The model under review builds one solid part; all positions refer to its coordinate system, in mm. Round coordinates to 2 decimals unless told otherwise and drop trailing zeros. Order: outer loops, then holes, each group sorted by start corner. A loop starts at its lowest first (then second) coordinate and runs counter-clockwise, first axis right, second up. Notation, with made-up numbers: (76, 49.5) - (84, 49.5) arc R14 cw to (84, 60.5) - close; hole circle Ø10 at (-2.75, -5). An arc over 180 degrees is marked (long way). One line per question, with ' | ' between items. Start each with the question number.
Item 1: Add section C-C on x = -2.5. State the section outline as (y, z) points.
Item 2: For L1, parallel to Z at x = -7.25, y = 20; L2, parallel to Z at x = -9.5, y = 20; L3, parallel to X at y = 25, z = 61, list the stretches that pass through material, from the lowest coordinate up. Write a range as [from, to].
Item 3: Add section D-D on z = -6. State the section outline as (x, y) points, and give its area (3 significant figures).
Item 4: Add section B-B on y = 12. State the section outline as (x, z) points, and give its area (3 significant figures).
Item 5: Add section A-A on y = 20. State the section outline as (x, z) points, and give its area (3 significant figures).
Item 6: Insertion check: pin 1 Ø3 at (x, y) = (-18, 15.5) entering from -Z; pin 2 Ø3 at (y, z) = (15, 62) entering from -X; pin 3 Ø10 at (x, y) = (-13, 34) entering from +Z; pin 4 Ø2.5 at (y, z) = (20, 11.74) entering from -X. Each pin has a flat end and moves straight along its axis. Give the tip position at first contact, or say it passes through.
Autodesk Inventor part; units mm, degrees
ref_plane "YZ Plane" through (0, 0, 0) normal (1, 0, 0) x (0, 1, 0)
ref_plane "XZ Plane" through (0, 0, 0) normal (0, 1, 0) x (-1, 0, 0)
ref_plane "XY Plane" through (0, 0, 0) normal (0, 0, 1) x (1, 0, 0)
sketch "Sketch1" plane through (0, 0, 0) normal (0, 1, 0) x (-1, 0, 0)
  line L0 (0.6887, 107.7362) -> (0.6887, -18.2638)
  line L1 (0.6887, -18.2638) -> (20.6887, 1.7362)
  line L2 (20.6887, 1.7362) -> (20.6887, 87.7362)
  line L3 (20.6887, 87.7362) -> (0.6887, 107.7362)
  point P0 (0, 0)
  dimension "d0" = 45
  dimension "d1" = 86
  dimension "d3" = 20
  dimension "d4" = 126
extrude "Extrusion1" add sketch "Sketch1" along normal blind 40
sketch "Sketch2" plane through (-20.6887, 0, 1.7362) normal (-1, 0, 0) x (0, 0, 1)
  line L0 (0, 0) -> (0, 40) construction
  line L1 (0, 20) -> (86, 20) construction
  line L2 (86, 0) -> (86, 40) construction
  line L3 (-20, 0) -> (-20, 40) construction
  line L4 (10, 20) -> (-20, 20) construction
  line L5 (76, 20) -> (106, 20) construction
  line L6 (106, 0) -> (106, 40) construction
  line L7 (22, 9.5) -> (28, 9.5)
  line L8 (28, 9.5) -> (28, 30.5)
  line L9 (28, 30.5) -> (22, 30.5)
  line L10 (22, 30.5) -> (22, 9.5)
  line L11 (43, 20) -> (43, 31.7658) construction
  line L12 (64, 9.5) -> (58, 9.5)
  line L13 (58, 9.5) -> (58, 30.5)
  line L14 (58, 30.5) -> (64, 30.5)
  line L15 (64, 30.5) -> (64, 9.5)
  point P0 (-1.7362, 0)
  point P1 (22, 20)
  dimension "d7" = 30
  dimension "d8" = 5
  dimension "d9" = 20
  dimension "d10" = 15
extrude "Extrusion2" cut sketch "Sketch2" against normal blind 4
hole "Hole1" at (-20.6887, 20, 11.7362) at (-20.6887, 20, 77.7362) direction (1, 0, 0) diameter 4 end through all countersink diameter 7 countersink angle 90
equation "\"d1\" = outer_carriage_innside_length"
equation "\"d3\" = outer_carriage_width"
equation "\"d5\" = outer_carriage_height"
equation "\"d7\" = outer_carriage_corner_to_screw"
equation "\"d8\" = glide_plate_width"
equation "\"d9\" = glide_plate_length"
equation "\"d10\" = outer_carriage_center_to_glideplate"
equation "\"d11\" = glide_plate_height - outer_carriage_to_centerlegg"
equation "\"d13\" = outer_carriage_screw_size"
equation "\"outer_carriage_length\" = d4"
equation "\"outer_carriage_height\" = 40"
equation "\"outer_carriage_width\" = 20"
equation "\"outer_carriage_screw_size\" = 4"
equation "\"outer_carriage_innside_length\" = long_centerlegg_width + 2 * outer_carriage_to_centerlegg"
equation "\"outer_carriage_center_to_glideplate\" = 15"
equation "\"outer_carriage_to_centerlegg\" = 1"
properties part number "01_one_side_base_model"
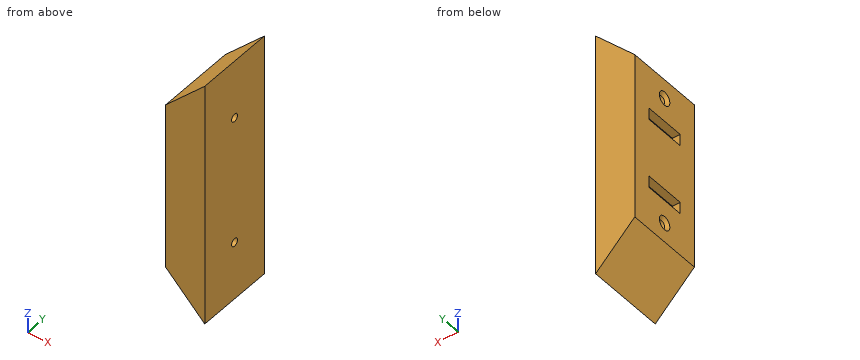
Determined:
1) outline: (0, -16.45) - (40, -16.45) - (40, 105.92) - (0, 105.92) - close; hole circle Ø4 at (20, 11.74); hole circle Ø4 at (20, 77.74)
2) L1: [-11.7, 9.74], [13.74, 75.74], [79.74, 101.17] | L2: [-9.45, 9.74], [13.74, 75.74], [79.74, 98.92] | L3: [-16.69, -0.69]
3) outline: (-12.95, 0) - (-0.69, 0) - (-0.69, 40) - (-12.95, 40) - close | area: 491 mm2
4) outline: (-20.69, 1.74) - (-0.69, -18.26) - (-0.69, 107.74) - (-20.69, 87.74) - (-20.69, 65.74) - (-16.69, 65.74) - (-16.69, 59.74) - (-20.69, 59.74) - (-20.69, 29.74) - (-16.69, 29.74) - (-16.69, 23.74) - (-20.69, 23.74) - close | area: 2,070 mm2
5) outline: (-20.69, 1.74) - (-0.69, -18.26) - (-0.69, 9.74) - (-19.19, 9.74) - (-20.69, 8.24) - close; (-20.69, 15.24) - (-19.19, 13.74) - (-0.69, 13.74) - (-0.69, 75.74) - (-19.19, 75.74) - (-20.69, 74.24) - (-20.69, 65.74) - (-16.69, 65.74) - (-16.69, 59.74) - (-20.69, 59.74) - (-20.69, 29.74) - (-16.69, 29.74) - (-16.69, 23.74) - (-20.69, 23.74) - close; (-20.69, 81.24) - (-19.19, 79.74) - (-0.69, 79.74) - (-0.69, 107.74) - (-20.69, 87.74) - close | area: 1,910 mm2
6) pin 1: z = -2.45 | pin 2: x = -16.69 | pin 3: z = 100.42 | pin 4: through
